```python
from build123d import *


# Read off the part's stored shape, not the designer's step: Revolve4
with BuildPart() as part:
    # Sketch2 → Revolve1 (revolve)
    with BuildSketch(Plane(origin=(0, 0, 0), x_dir=(1, 0, 0), z_dir=(0, 1, 0)), mode=Mode.PRIVATE) as revolve1_sk:
        with BuildLine():
            Line((0, 88.9), (-23.467681094, 88.9))
            Line((-23.467681094, 88.9), (-23.467681094, 0))
            Line((-23.467681094, 0), (-8.405449734, -26.088549992))
            ThreePointArc((-8.405449734, -26.088549992), (-8.081511216, -27.07075529), (-8.175988072, -28.10067642))
            Line((-8.175988072, -28.10067642), (-27.000254561, -89.717228424))
            Line((-27.000254561, -89.717228424), (0, -89.717228424))
            Line((0, -89.717228424), (0, 88.9))
        make_face()
    revolve(revolve1_sk.sketch.rotate(Axis((0, 0, 0), (0, 0, -1)), 180), axis=Axis((0, 0, 0), (0, 0, -1)))

    # Revolve4 outline → Revolve4 (revolve)
    with BuildSketch(Plane.XZ):
        with BuildLine():
            Line((23.467681094, -88.9), (26.007681094, -88.9))
            Line((26.007681094, -88.9), (26.007681094, 0.680590949))
            Line((26.007681094, 0.680590949), (11.157211277, 26.402359187))
            ThreePointArc((11.157211277, 26.402359187), (10.83327276, 27.384564486), (10.927749616, 28.414485616))
            Line((10.927749616, 28.414485616), (29.656145308, 89.717228424))
            Line((29.656145308, 89.717228424), (27.000254561, 89.717228424))
            Line((27.000254561, 89.717228424), (8.175988072, 28.10067642))
            ThreePointArc((8.175988072, 28.10067642), (8.081511216, 27.07075529), (8.405449734, 26.088549992))
            Line((8.405449734, 26.088549992), (23.467681094, 0))
            Line((23.467681094, 0), (23.467681094, -88.9))
        make_face()
    revolve(axis=Axis((0, 0, 0), (0, 0, 1)))

    # Sketch6 → Cut-Revolve2 (revolve, cut)
    with BuildSketch(Plane(origin=(0, 0, 0), x_dir=(1, 0, 0), z_dir=(0, 1, 0)), mode=Mode.PRIVATE) as cut_revolve2_sk:
        with BuildLine():
            Line((0, 88.9), (-23.467681094, 88.9))
            Line((-23.467681094, 88.9), (-23.467681094, 0))
            Line((-23.467681094, 0), (-8.405449734, -26.088549992))
            ThreePointArc((-8.405449734, -26.088549992), (-8.081511216, -27.07075529), (-8.175988072, -28.10067642))
            Line((-8.175988072, -28.10067642), (-27.000254561, -89.717228424))
            Line((-27.000254561, -89.717228424), (0, -89.717228424))
            Line((0, -89.717228424), (0, 88.9))
        make_face()
    revolve(cut_revolve2_sk.sketch.rotate(Axis((0, 0, 98.648089845), (0, 0, -1)), 180), axis=Axis((0, 0, 98.648089845), (0, 0, -1)), mode=Mode.SUBTRACT)


solid = part.part
```
Geometry check sheet. Reference: the model listing, model coordinates, mm. A direction names the side the tool comes from. Round coordinates to 2 decimals unless told otherwise and drop trailing zeros. Order: outer loops, then holes, each group sorted by start corner. A loop starts at its lowest first (then second) coordinate and runs counter-clockwise, first axis right, second up. Notation, with made-up numbers: M 13.5,5.5 L 60.5,5.5 A16 cw 60.5,27.5 Z; hole C 61,43 d10. An arc over 180 degrees is marked long. Answer as CSV lines item,"result".
1) Sectioned sample at D-D on z = 66. Record the cut outline in (x, y), and give its area (3 significant figures).
Entries:
outline,"C 0,0 d44.82; hole C 0,0 d39.51"
area,"352 mm2"
2) Gauge pin test, flat ends, axial feed: pin 1 Ø2 at (y, z) = (-5, 37.5) entering from +X; pin 2 Ø5 at (x, z) = (-5, 27.5) entering from +Y; pin 3 Ø2 at (y, z) = (9, -10.5) entering from +X. Record the tip position at first contact, or that the pin passes through.
Entries:
pin 1,"x = 13.24"
pin 2,"y = 11.16"
pin 3,"x = 24.75"
3) Sectioned sample at A-A on y = 0. Record the cut outline in (x, z), and give its area (3 significant figures).
Entries:
outline,"M -29.66,89.72 L -10.93,28.41 A2.54 cw -11.16,26.4 L -26.01,0.68 L -26.01,-88.9 L -23.47,-88.9 L -23.47,0 L -8.41,26.09 A2.54 ccw -8.18,28.1 L -27,89.72 Z; M 8.18,28.1 A2.54 ccw 8.41,26.09 L 23.47,0 L 23.47,-88.9 L 26.01,-88.9 L 26.01,0.68 L 11.16,26.4 A2.54 cw 10.93,28.41 L 29.66,89.72 L 27,89.72 Z"
area,"943 mm2"
4) Tool access check on faces 1 (the face through (-5.64, -25.39, -43.48)), 2 (the face through (17.495, 5.509, 52.684)), 3 (the face through (13, -24, 89.717)). Record the directions out of +Z, -Z, +X, -X, +Y, -Y that give a thin tool (end or side, any length) a straight path to the whole face; none if there is none.
Entries:
face 1,"-Z"
face 2,"none"
face 3,"+Z, +X, -X, +Y, -Y"
5) Sectioned sample at C-C on z = -26. Record the cut outline in (x, y).
Entries:
outline,"C 0,0 d52.02; hole C 0,0 d46.94"
6) Thickness scan on probe 1 along Y at (x, z) = (0, -20); probe 2 along X at (y, z) = (-23.5, -71); probe 3 along Y at (x, z) = (7, -22). Record the ranges inside material, lowest first. Write a range as [from, to].
Entries:
probe 1,"[-26.01, -23.47], [23.47, 26.01]"
probe 2,"[-11.14, 11.14]"
probe 3,"[-25.05, -22.4], [22.4, 25.05]"
7) Mould release check, pull along Y, two halves, no side actions. Record for faces 4 (the face through (-2.933, -13.207, 22.295)), 5 (the face through (14.907, -4.694, 52.494)), 6 (the face through (-2.71, 12.19, 19.02)), 7 (the face through (13.6, 19.4, -88.9)): +Y half, -Y half, draft (parallel to the pull), parting line (faces both ways), or undercut.
Entries:
face 4,"parting line"
face 5,"undercut"
face 6,"undercut"
face 7,"draft"
